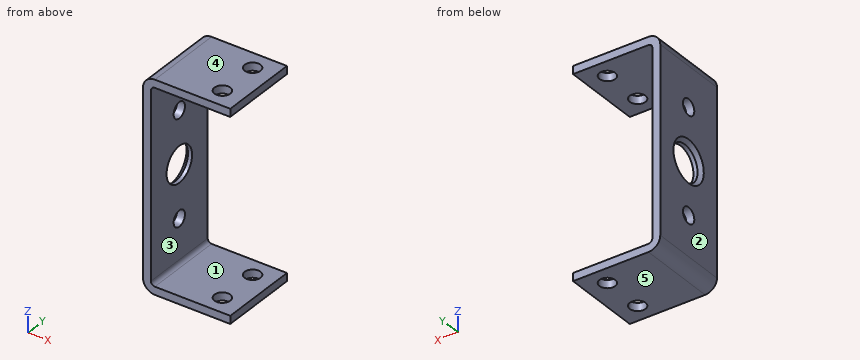
from build123d import *

# Parameters (mm, degrees)
BRIDA_BASE2_DEPTH                       = 7.5
CROQUIS10_R                             = 1.5
CORTAR_EXTRUIR1_DEPTH                   = 43.774671244
CORTAR_EXTRUIR2_REACH                   = 27.853
CROQUIS13_R                             = 1.5
TALADRO_DE_MARGEN_PARA_1_41_D           = 6.7564
TALADRO_DE_MARGEN_PARA_1_41_DEPTH       = 3.65
TALADRO_DE_MARGEN_PARA_1_41_CSINK_D     = 8.0264
TALADRO_DE_MARGEN_PARA_1_41_CSINK_ANGLE = 82
TALADRO_DE_MARGEN_PARA_1_41_TIP         = 2.029827343


# Sheet-metal steps are written as plain solids
with BuildPart() as part:
    # Croquis1 → Brida base2 (new, symmetric)
    with BuildSketch(Plane(origin=(122.052362923, 0, 0), x_dir=(1, 0, 0), z_dir=(0, 1, 0))):
        with BuildLine():
            Line((-107.052362923, 18.175), (-121.315762923, 18.175))
            ThreePointArc((-121.315762923, 18.175), (-121.836617778, 17.959254855), (-122.052362923, 17.4384))
            Line((-122.052362923, 17.4384), (-122.052362923, -17.4384))
            ThreePointArc((-122.052362923, -17.4384), (-121.836617778, -17.959254855), (-121.315762923, -18.175))
            Line((-121.315762923, -18.175), (-107.052362923, -18.175))
            Line((-107.052362923, -18.175), (-107.052362923, -19.675))
            Line((-107.052362923, -19.675), (-121.315762923, -19.675))
            ThreePointArc((-121.315762923, -19.675), (-122.89727795, -19.019915027), (-123.552362923, -17.4384))
            Line((-123.552362923, -17.4384), (-123.552362923, 17.4384))
            ThreePointArc((-123.552362923, 17.4384), (-122.89727795, 19.019915027), (-121.315762923, 19.675))
            Line((-121.315762923, 19.675), (-107.052362923, 19.675))
            Line((-107.052362923, 19.675), (-107.052362923, 18.175))
        make_face()
    extrude(amount=BRIDA_BASE2_DEPTH, both=True)

    # Croquis10 → Cortar-Extruir1 (cut, through all)
    with BuildSketch(Plane(origin=(0, 0, -19.675), x_dir=(-1, 0, 0), z_dir=(0, 0, -1))):
        with Locations((-11, 4)):
            Circle(CROQUIS10_R)
        with Locations((-11, -4)):
            Circle(CROQUIS10_R)
    extrude(amount=-CORTAR_EXTRUIR1_DEPTH, mode=Mode.SUBTRACT)

    # Croquis13 → Cortar-Extruir2 (cut, up to next)
    with BuildSketch(Plane(origin=(0, 0, 0), x_dir=(0, 0, 1), z_dir=(1, 0, 0)), mode=Mode.PRIVATE) as cortar_extruir2_sk1:
        with Locations(Location((-9.9, 0, 0), (0, 0, 270))):
            Circle(CROQUIS13_R)
    cortar_extruir2_tool1 = extrude(cortar_extruir2_sk1.sketch, amount=-CORTAR_EXTRUIR2_REACH, mode=Mode.PRIVATE) & part.part
    # Croquis13 → Cortar-Extruir2 (cut, up to next)
    with BuildSketch(Plane(origin=(0, 0, 0), x_dir=(0, 0, 1), z_dir=(1, 0, 0)), mode=Mode.PRIVATE) as cortar_extruir2_sk2:
        with Locations(Location((9.9, 0, 0), (0, 0, 270))):
            Circle(CROQUIS13_R)
    cortar_extruir2_tool2 = extrude(cortar_extruir2_sk2.sketch, amount=-CORTAR_EXTRUIR2_REACH, mode=Mode.PRIVATE) & part.part
    add(cortar_extruir2_tool1.solids().sort_by_distance((0, 0, -9.9))[0], mode=Mode.SUBTRACT)
    add(cortar_extruir2_tool2.solids().sort_by_distance((0, 0, 9.9))[0], mode=Mode.SUBTRACT)

    # Taladro de margen para 1/41
    with Locations(Plane.ZY.offset(1.5)):
        with Locations((0, 0)):
            CounterSinkHole(TALADRO_DE_MARGEN_PARA_1_41_D / 2, TALADRO_DE_MARGEN_PARA_1_41_CSINK_D / 2, depth=TALADRO_DE_MARGEN_PARA_1_41_DEPTH, counter_sink_angle=TALADRO_DE_MARGEN_PARA_1_41_CSINK_ANGLE)
            with Locations((0, 0, -(TALADRO_DE_MARGEN_PARA_1_41_DEPTH + TALADRO_DE_MARGEN_PARA_1_41_TIP / 2))):  # 118° drill point
                Cone(0, TALADRO_DE_MARGEN_PARA_1_41_D / 2, TALADRO_DE_MARGEN_PARA_1_41_TIP, mode=Mode.SUBTRACT)


solid = part.part
Can you work these out from the model? Positions are in its coordinate system, mm. Face numbers are marked on the shaded views. A direction names the side the tool comes from. Coordinates: 2 decimals unless noted, no trailing zeros. Order: outer loops, then holes, each group sorted by start corner. A loop starts at its lowest first (then second) coordinate and runs counter-clockwise, first axis right, second up. Notation, with made-up numbers: M 68,-38.75 L 100,-38.75 A15 cw 100,-9.75 Z; hole C 2,58 d10. An arc over 180 degrees is marked long. Write item = value, one per line.
(1) Suppose I cut it at D-D on x = 11. Please give me the cut outline in (y, z) (3 decimals), plus the area to 3 significant figures.
Results are:
outline = M -7.5,-19.675 L -5.5,-19.675 L -5.5,-18.175 L -7.5,-18.175 Z; M -7.5,18.175 L -5.5,18.175 L -5.5,19.675 L -7.5,19.675 Z; M -2.5,-19.675 L 2.5,-19.675 L 2.5,-18.175 L -2.5,-18.175 Z; M -2.5,18.175 L 2.5,18.175 L 2.5,19.675 L -2.5,19.675 Z; M 5.5,-19.675 L 7.5,-19.675 L 7.5,-18.175 L 5.5,-18.175 Z; M 5.5,18.175 L 7.5,18.175 L 7.5,19.675 L 5.5,19.675 Z
area = 27.0 mm2
(2) If we mould it in two halves opening along Z, with no side actions, what happens to the marked faces 3, 4 and 5? For each: pulls with the +Z half, pulls with the -Z half, needs draft (parallel to the pull), parting line crosses it, or undercut.
Results are:
face_3 = undercut
face_4 = pulls with the +Z half
face_5 = pulls with the -Z half
(3) Suppose I cut it at C-C on y = -6.25. Please give me the cut outline in (x, z) (3 decimals).
Results are:
outline = M -1.5,-17.438 A2.237 ccw 0.737,-19.675 L 15,-19.675 L 15,-18.175 L 0.737,-18.175 A0.737 cw 0,-17.438 L 0,17.438 A0.737 cw 0.737,18.175 L 15,18.175 L 15,19.675 L 0.737,19.675 A2.237 ccw -1.5,17.438 Z
(4) Suppose I cut it at B-B on x = 8.5. Please give me the cut outline in (y, z) (3 decimals), plus the area to 3 significant figures.
Results are:
outline = M -7.5,-19.675 L 7.5,-19.675 L 7.5,-18.175 L -7.5,-18.175 Z; M -7.5,18.175 L 7.5,18.175 L 7.5,19.675 L -7.5,19.675 Z
area = 45.0 mm2
(5) For pin 1 Ø8 at (y, z) = (0, 0) entering from +X, with a flat end and sliding along its axis, tell me the tip position at first contact or that it passes through.
Results are:
pin_1 = 0
(6) For the marked faces 1 and 2, which set-ups out of +Z, -Z, +X, -X, +Y, -Y let a thin tool reach every point of the face, with its end or its side?
Results are:
face_1 = +X, +Y, -Y
face_2 = +Z, -Z, -X, +Y, -Y
(7) I need wall thicknesses on line 1 along Y through (x, z) = (11, -18.85); line 2 along Z through (x, y) = (-0.55, 0); line 3 along Z through (x, y) = (1, 5.25) (3 decimals). Which ranges of each line are inside material? Lowest first, please. Write a range as [from, to].
Results are:
line_1 = [-7.5, -5.5], [-2.5, 2.5], [5.5, 7.5]
line_2 = [-19.27, -11.4], [-8.4, -3.38], [3.38, 8.4], [11.4, 19.27]
line_3 = [-19.675, -18.175], [18.175, 19.675]
(8) Suppose I cut it at A-A on z = -9.9. Please give me the cut outline in (x, y).
Results are:
outline = M -1.5,-7.5 L 0,-7.5 L 0,-1.5 L -1.5,-1.5 Z; M -1.5,1.5 L 0,1.5 L 0,7.5 L -1.5,7.5 Z
